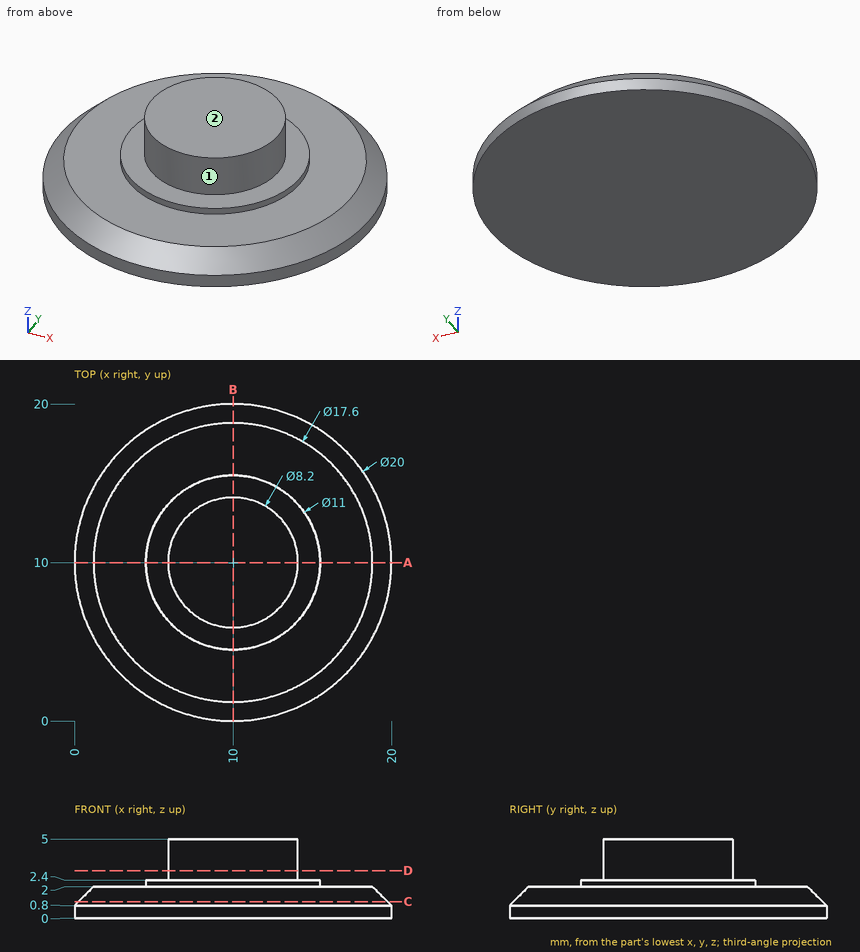
Print and shaded views of the part. All mm, measured from the part's lowest x, y and z. A direction names the side the tool comes from. Give positions to 0.01 mm unless a question says otherwise; leave off trailing zeros. Write each loop counter-clockwise with the first axis right and the second up, starting at its lowest first coordinate (ties: lowest second). Pieces come first, ordered by that corner, then holes. Notation, with made-up numbers: (65.5, -27.5) - (111.5, -27.5) arc R29 cw to (111.5, -2.5) - close; hole circle Ø6 at (72.25, 63). An arc over 180 degrees is marked (long way). Put each result on its own line as item: value.
(1) Wall check: L1, parallel to Z at x = 9, y = 1.5; L2, parallel to Z at x = 4.75, y = 10.5; L3, parallel to Y at x = 10, z = 4.25. Give the ranges that are in metal, low to high.
Working result:
L1: 0 to 2
L2: 0 to 2.4
L3: 5.9 to 14.1
(2) Saw through at C-C (z = 1.05). List the corners of the cut face in (x, y).
Working result:
outline: circle Ø19.5 at (10, 10)
(3) Saw through at D-D (z = 3). List the corners of the cut face in (x, y), then the cut area to 3 significant figures.
Working result:
outline: circle Ø8.2 at (10, 10)
area: 52.8 mm^2
(4) Saw through at A-A (y = 10). List the corners of the cut face in (x, z), then the cut area to 3 significant figures.
Working result:
outline: (0, 0) - (20, 0) - (20, 0.8) - (18.8, 2) - (15.5, 2) - (15.5, 2.4) - (14.1, 2.4) - (14.1, 5) - (5.9, 5) - (5.9, 2.4) - (4.5, 2.4) - (4.5, 2) - (1.2, 2) - (0, 0.8) - close
area: 64.3 mm^2
(5) Drop a flat-ended pin along its axis: pin 1 Ø3 at (y, z) = (17.5, 4) entering from +X. Give the stop position or say it passes through.
Working result:
pin 1: through
(6) Tool access for the marked faces 1 and 2: list every direction of +Z, -Z, +X, -X, +Y, -Y with a clear straight run to the whole face (end or side of a thin tool).
Working result:
face 1: +Z
face 2: +Z, +X, -X, +Y, -Y
